Geometry: final body of the model. Coordinates: model frame, mm. Face numbers are marked on the shaded views. A direction names the side the tool comes from. Give positions to 0.01 mm unless a question says otherwise; leave off trailing zeros. Loops run counter-clockwise (first coordinate to the right, second up) from the corner with the lowest first, then second, coordinate; pieces in that order, holes last. Notation, with made-up numbers: M -6.75,61.5 L 20.25,61.5 A24 cw 20.25,87.5 Z; hole C 27,45.25 d3. An arc over 180 degrees is marked long. Put each result on its own line as item: value.
```python
from build123d import *

# Parameters (mm, degrees)
F0_R     = 11.049
F1_DEPTH = 25.4
F2_DEPTH = 25.4


with BuildPart() as f1:
    # F0 (on Top) → F1 (new body)
    with BuildSketch(Plane.XY):
        with BuildLine():
            ThreePointArc((11.7814514995, 7.5072165658), (13.4117071517, 3.9098607745), (13.97, 0))
            ThreePointArc((13.97, 0), (-3.3198148199, -13.5698094888), (-12.3921660074, 6.4494280091))
            ThreePointArc((-12.3921660074, 6.4494280091), (-18.1144161616, 5.491925307), (-22.3375658393, 9.4701114579))
            ThreePointArc((-22.3375658393, 9.4701114579), (-19.1125242771, 17.0828384763), (-13.1982271537, 22.86))
            ThreePointArc((-13.1982271537, 22.86), (-15.0773857713, 28.2596310433), (-14.8345973958, 33.9717502926))
            ThreePointArc((-14.8345973958, 33.9717502926), (-27.1350680748, 15.1641790656), (-37.4838164006, -4.7839968529))
            ThreePointArc((-37.4838164006, -4.7839968529), (-20.7712342362, -1.076155213), (-11.1564543073, -15.24))
            ThreePointArc((-11.1564543073, -15.24), (-14.1650946399, -24.3312837754), (-22.0031000665, -29.8330133459))
            ThreePointArc((-22.0031000665, -29.8330133459), (0.4349697391, -31.081747819), (22.8849710065, -30.0699388073))
            ThreePointArc((22.8849710065, -30.0699388073), (11.2593167407, -13.4723274374), (26.3964543073, 0))
            ThreePointArc((26.3964543073, 0), (24.3504342278, 8.0105123163), (19.3701400189, 14.6098437466))
            ThreePointArc((19.3701400189, 14.6098437466), (13.8133549124, 12.9415819171), (11.7814514995, 7.5072165658))
        make_face()
        with BuildLine():
            ThreePointArc((15.2189978183, 17.4838557876), (17.3812836494, 16.1720980867), (19.3701400189, 14.6098437466))
            ThreePointArc((19.3701400189, 14.6098437466), (24.3504342278, 8.0105123163), (26.3964543073, 0))
            ThreePointArc((26.3964543073, 0), (32.0122512707, -1.0724164211), (36.8376974623, -4.1387369467))
            ThreePointArc((36.8376974623, -4.1387369467), (26.7000983357, 15.9175687534), (14.5988453941, 34.8539356602))
            ThreePointArc((14.5988453941, 34.8539356602), (15.0788594364, 32.69033891), (15.24, 30.48))
            ThreePointArc((15.24, 30.48), (14.6051180743, 26.1270554752), (12.7533692867, 22.1367888773))
            ThreePointArc((12.7533692867, 22.1367888773), (17.57558266, 21.7123752268), (15.2189978183, 17.4838557876))
        make_face()
        with BuildLine():
            ThreePointArc((-13.1982271537, 22.86), (-7.62, 17.2817728463), (0, 15.24))
            ThreePointArc((0, 15.24), (7.2493814388, 17.074625378), (12.7533692867, 22.1367888773))
            ThreePointArc((12.7533692867, 22.1367888773), (14.6051180743, 26.1270554752), (15.24, 30.48))
            ThreePointArc((15.24, 30.48), (15.0788594364, 32.69033891), (14.5988453941, 34.8539356602))
            ThreePointArc((14.5988453941, 34.8539356602), (11.505690551, 39.090096987), (8.3139361742, 43.2524729513))
            ThreePointArc((8.3139361742, 43.2524729513), (-5.6712175905, 44.6254901308), (-14.8345973958, 33.9717502926))
            ThreePointArc((-14.8345973958, 33.9717502926), (-15.0773857713, 28.2596310433), (-13.1982271537, 22.86))
        make_face()
        with BuildLine():
            ThreePointArc((11.049, 30.48), (7.8128228253, 22.6671771747), (0, 19.431))
            ThreePointArc((0, 19.431), (-7.8128228253, 38.2928228253), (11.049, 30.48))
        make_face(mode=Mode.SUBTRACT)
        with BuildLine():
            ThreePointArc((36.8376974623, -4.1387369467), (32.0122512707, -1.0724164211), (26.3964543073, 0))
            ThreePointArc((26.3964543073, 0), (11.2593167407, -13.4723274374), (22.8849710065, -30.0699388073))
            ThreePointArc((22.8849710065, -30.0699388073), (28.1001717516, -29.5092687987), (33.3007722652, -28.8263164079))
            ThreePointArc((33.3007722652, -28.8263164079), (39.3864390202, -23.2098116139), (41.6364543073, -15.24))
            ThreePointArc((41.6364543073, -15.24), (40.3854168436, -9.1929736928), (36.8376974623, -4.1387369467))
        make_face()
        with Locations((26.3964543073, -15.24)):
            Circle(F0_R, mode=Mode.SUBTRACT)
        with BuildLine():
            ThreePointArc((33.3007722652, -28.8263164079), (28.1001717516, -29.5092687987), (22.8849710065, -30.0699388073))
            ThreePointArc((22.8849710065, -30.0699388073), (28.2032417659, -30.3725185967), (33.3007722652, -28.8263164079))
        make_face()
        with BuildLine():
            ThreePointArc((8.3139361742, 43.2524729513), (11.505690551, 39.090096987), (14.5988453941, 34.8539356602))
            ThreePointArc((14.5988453941, 34.8539356602), (12.2017517987, 39.6109831367), (8.3139361742, 43.2524729513))
        make_face()
        with BuildLine():
            ThreePointArc((-41.6147084394, -14.4261565433), (-35.8111993144, -27.2241635692), (-22.0031000665, -29.8330133459))
            ThreePointArc((-22.0031000665, -29.8330133459), (-14.1650946399, -24.3312837754), (-11.1564543073, -15.24))
            ThreePointArc((-11.1564543073, -15.24), (-20.7712342362, -1.076155213), (-37.4838164006, -4.7839968529))
            ThreePointArc((-37.4838164006, -4.7839968529), (-39.6058623026, -9.5808281882), (-41.6147084394, -14.4261565433))
        make_face()
        with Locations((-26.3964543073, -15.24)):
            Circle(F0_R, mode=Mode.SUBTRACT)
        with BuildLine():
            ThreePointArc((-41.6147084394, -14.4261565433), (-39.6058623026, -9.5808281882), (-37.4838164006, -4.7839968529))
            ThreePointArc((-37.4838164006, -4.7839968529), (-40.4049935646, -9.23846454), (-41.6147084394, -14.4261565433))
        make_face()
    extrude(amount=F1_DEPTH)

    # F0 (on Top) → F2 (join)
    with BuildSketch(Plane.XY):
        with BuildLine():
            ThreePointArc((11.7814514995, 7.5072165658), (13.4117071517, 3.9098607745), (13.97, 0))
            ThreePointArc((13.97, 0), (-3.3198148199, -13.5698094888), (-12.3921660074, 6.4494280091))
            ThreePointArc((-12.3921660074, 6.4494280091), (-18.1144161616, 5.491925307), (-22.3375658393, 9.4701114579))
            ThreePointArc((-22.3375658393, 9.4701114579), (-19.1125242771, 17.0828384763), (-13.1982271537, 22.86))
            ThreePointArc((-13.1982271537, 22.86), (-15.0773857713, 28.2596310433), (-14.8345973958, 33.9717502926))
            ThreePointArc((-14.8345973958, 33.9717502926), (-27.1350680748, 15.1641790656), (-37.4838164006, -4.7839968529))
            ThreePointArc((-37.4838164006, -4.7839968529), (-20.7712342362, -1.076155213), (-11.1564543073, -15.24))
            ThreePointArc((-11.1564543073, -15.24), (-14.1650946399, -24.3312837754), (-22.0031000665, -29.8330133459))
            ThreePointArc((-22.0031000665, -29.8330133459), (0.4349697391, -31.081747819), (22.8849710065, -30.0699388073))
            ThreePointArc((22.8849710065, -30.0699388073), (11.2593167407, -13.4723274374), (26.3964543073, 0))
            ThreePointArc((26.3964543073, 0), (24.3504342278, 8.0105123163), (19.3701400189, 14.6098437466))
            ThreePointArc((19.3701400189, 14.6098437466), (13.8133549124, 12.9415819171), (11.7814514995, 7.5072165658))
        make_face()
        with BuildLine():
            ThreePointArc((15.2189978183, 17.4838557876), (17.3812836494, 16.1720980867), (19.3701400189, 14.6098437466))
            ThreePointArc((19.3701400189, 14.6098437466), (24.3504342278, 8.0105123163), (26.3964543073, 0))
            ThreePointArc((26.3964543073, 0), (32.0122512707, -1.0724164211), (36.8376974623, -4.1387369467))
            ThreePointArc((36.8376974623, -4.1387369467), (26.7000983357, 15.9175687534), (14.5988453941, 34.8539356602))
            ThreePointArc((14.5988453941, 34.8539356602), (15.0788594364, 32.69033891), (15.24, 30.48))
            ThreePointArc((15.24, 30.48), (14.6051180743, 26.1270554752), (12.7533692867, 22.1367888773))
            ThreePointArc((12.7533692867, 22.1367888773), (17.57558266, 21.7123752268), (15.2189978183, 17.4838557876))
        make_face()
        with BuildLine():
            ThreePointArc((-13.1982271537, 22.86), (-7.62, 17.2817728463), (0, 15.24))
            ThreePointArc((0, 15.24), (7.2493814388, 17.074625378), (12.7533692867, 22.1367888773))
            ThreePointArc((12.7533692867, 22.1367888773), (14.6051180743, 26.1270554752), (15.24, 30.48))
            ThreePointArc((15.24, 30.48), (15.0788594364, 32.69033891), (14.5988453941, 34.8539356602))
            ThreePointArc((14.5988453941, 34.8539356602), (11.505690551, 39.090096987), (8.3139361742, 43.2524729513))
            ThreePointArc((8.3139361742, 43.2524729513), (-5.6712175905, 44.6254901308), (-14.8345973958, 33.9717502926))
            ThreePointArc((-14.8345973958, 33.9717502926), (-15.0773857713, 28.2596310433), (-13.1982271537, 22.86))
        make_face()
        with BuildLine():
            ThreePointArc((11.049, 30.48), (7.8128228253, 22.6671771747), (0, 19.431))
            ThreePointArc((0, 19.431), (-7.8128228253, 38.2928228253), (11.049, 30.48))
        make_face(mode=Mode.SUBTRACT)
        with BuildLine():
            ThreePointArc((36.8376974623, -4.1387369467), (32.0122512707, -1.0724164211), (26.3964543073, 0))
            ThreePointArc((26.3964543073, 0), (11.2593167407, -13.4723274374), (22.8849710065, -30.0699388073))
            ThreePointArc((22.8849710065, -30.0699388073), (28.1001717516, -29.5092687987), (33.3007722652, -28.8263164079))
            ThreePointArc((33.3007722652, -28.8263164079), (39.3864390202, -23.2098116139), (41.6364543073, -15.24))
            ThreePointArc((41.6364543073, -15.24), (40.3854168436, -9.1929736928), (36.8376974623, -4.1387369467))
        make_face()
        with Locations((26.3964543073, -15.24)):
            Circle(F0_R, mode=Mode.SUBTRACT)
        with BuildLine():
            ThreePointArc((33.3007722652, -28.8263164079), (28.1001717516, -29.5092687987), (22.8849710065, -30.0699388073))
            ThreePointArc((22.8849710065, -30.0699388073), (28.2032417659, -30.3725185967), (33.3007722652, -28.8263164079))
        make_face()
        with BuildLine():
            ThreePointArc((8.3139361742, 43.2524729513), (11.505690551, 39.090096987), (14.5988453941, 34.8539356602))
            ThreePointArc((14.5988453941, 34.8539356602), (12.2017517987, 39.6109831367), (8.3139361742, 43.2524729513))
        make_face()
        with BuildLine():
            ThreePointArc((-41.6147084394, -14.4261565433), (-35.8111993144, -27.2241635692), (-22.0031000665, -29.8330133459))
            ThreePointArc((-22.0031000665, -29.8330133459), (-14.1650946399, -24.3312837754), (-11.1564543073, -15.24))
            ThreePointArc((-11.1564543073, -15.24), (-20.7712342362, -1.076155213), (-37.4838164006, -4.7839968529))
            ThreePointArc((-37.4838164006, -4.7839968529), (-39.6058623026, -9.5808281882), (-41.6147084394, -14.4261565433))
        make_face()
        with Locations((-26.3964543073, -15.24)):
            Circle(F0_R, mode=Mode.SUBTRACT)
        with BuildLine():
            ThreePointArc((-41.6147084394, -14.4261565433), (-39.6058623026, -9.5808281882), (-37.4838164006, -4.7839968529))
            ThreePointArc((-37.4838164006, -4.7839968529), (-40.4049935646, -9.23846454), (-41.6147084394, -14.4261565433))
        make_face()
    extrude(amount=F2_DEPTH)


solid = f1.part
```
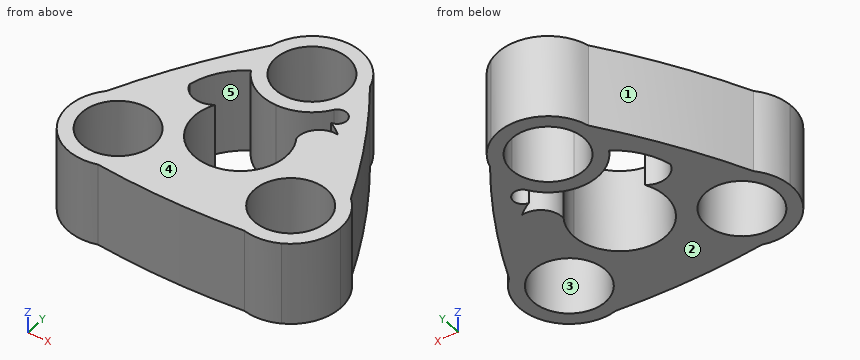
Item 1: Mould query, pull axis Y, two halves, no side actions, for the marked faces 1, 2 and 3. Classes: pulls with the +Y half, pulls with the -Y half, needs draft (parallel to the pull), parting line crosses it, or undercut.
Output values:
face 1: pulls with the +Y half
face 2: needs draft
face 3: undercut
Item 2: Line query: probe 1 along X at (y, z) = (-25, 24); probe 2 along Y at (x, z) = (-3, 13.5); probe 3 along X at (y, z) = (-19.5, 16). Output: solid intervals per line, ascending. Write a range as [from, to].
Output values:
probe 1: [-38.1, -31.58], [-21.22, 21.22], [31.58, 38.1]
probe 2: [-31.04, -13.64], [15.54, 19.85], [41.11, 45.42]
probe 3: [-41.03, -36.59], [-16.2, 16.2], [36.59, 41.03]
Item 3: Set-up query: the marked faces 4 and 5. Return all of +Z, -Z, +X, -X, +Y, -Y with unobstructed straight access to the full face (end or side cutting, diameter ignored); none if empty.
Output values:
face 4: +Z, +X, -X, +Y, -Y
face 5: +Z, -Z
Item 4: Section C-C on y = -20. Output: boundary loops of the cut face in (x, z).
Output values:
outline: M -40.87,0 L -36.37,0 L -36.37,25.4 L -40.87,25.4 Z; M -16.43,0 L 16.43,0 L 16.43,25.4 L -16.43,25.4 Z; M 36.37,0 L 40.87,0 L 40.87,25.4 L 36.37,25.4 Z
Item 5: Section D-D on x = -8.5. Output: boundary loops of the cut face in (y, z), then the cut area to 3 significant figures.
Output values:
outline: M -30.86,0 L -11.09,0 L -11.09,25.4 L -30.86,25.4 Z; M 17.83,0 L 23.42,0 L 23.42,25.4 L 17.83,25.4 Z; M 37.54,0 L 43.13,0 L 43.13,25.4 L 37.54,25.4 Z
area: 786 mm²
Item 6: Section A-A on x = 30.5. Output: boundary loops of the cut face in (y, z).
Output values:
outline: M -29.92,0 L -25.5,0 L -25.5,25.4 L -29.92,25.4 Z; M -4.98,0 L 8.97,0 L 8.97,25.4 L -4.98,25.4 Z
Item 7: Pin query (flat end, axial travel): pin 1 Ø1 at (x, z) = (-12.5, 20.5) entering from +Y; pin 2 Ø1 at (y, z) = (20.5, 8.5) entering from -X; pin 3 Ø12 at (y, z) = (18.5, 13) entering from +X; pin 4 Ø1.5 at (x, y) = (15, 33) entering from -Z. Return the tip coordinate at first contact, or that it passes through.
Output values:
pin 1: y = 39.87
pin 2: x = -24.23
pin 3: x = 28.61
pin 4: z = 0
Item 8: Section B-B on y = 32.5. Output: boundary loops of the cut face in (x, z), then the cut area to 3 significant figures.
Output values:
outline: M -15.9,0 L -10.86,0 L -10.86,25.4 L -15.9,25.4 Z; M 10.86,0 L 16.25,0 L 16.25,25.4 L 10.86,25.4 Z
area: 265 mm²
